Check sheet for the modelled part. Datum: model origin and axes. Units: mm. Face numbers are marked on the shaded views. A direction names the side the tool comes from. Give positions to 0.01 mm unless a question says otherwise; leave off trailing zeros. Order: outer loops, then holes, each group sorted by start corner. A loop starts at its lowest first (then second) coordinate and runs counter-clockwise, first axis right, second up.
Item 1: Access from +Z, -Z, +X, -X, +Y, -Y to the whole of each face (thin tool, end or side, straight path). Record for the marked faces 5, 6, 7, 8 and 9.
Item 2: Sectioned sample at D-D on y = -6. Record the boundary of the cut face in (x, z).
Item 3: Sectioned sample at A-A on y = -8.5. Record the boundary of the cut face in (x, z), and give its area (3 significant figures).
Item 4: Gauge pin test, flat ends, axial feed: P1, Ø6.5, axis at x = -14.5, z = 1, coming from the +Y side; P2, Ø2.5, axis at x = 0, z = -6, coming from the -Y side; P3, Ø6.5, axis at y = -4, z = -0.5, coming from the +X side; P4, Ø0.6, axis at y = 1, z = -4.5, coming from the -X side. Record the tip position at first contact, or that the pin passes through.
Item 5: Material ranges on line 1 along X through (y, z) = (-9.15, 0); line 2 along Z through (x, y) = (0, 0.45); line 3 along Y through (x, z) = (11.5, 1.5), recorded low to high.
Item 6: Sectioned sample at B-B on z = 0. Record the boundary of the cut face in (x, y), and give its area (3 significant figures).
Item 7: Release check for a two-part mould opening along X. For the marked faces 1, 2, 3 and 4 record: released by +X, released by -X, zero draft, split by the parting line, or undercut.
Item 8: Sectioned sample at C-C on x = 0. Record the boundary of the cut face in (y, z).
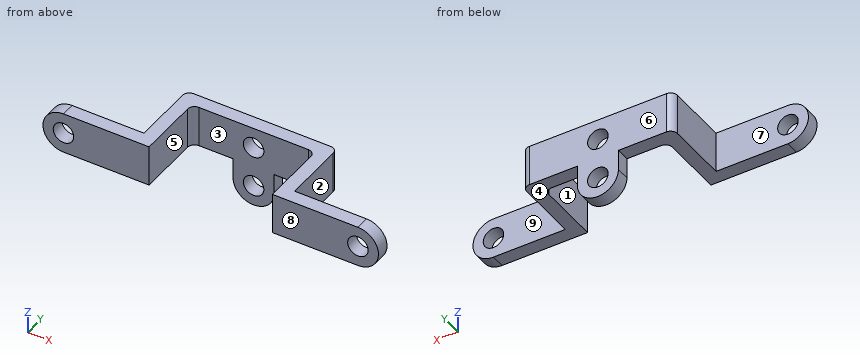
Autodesk Inventor part; units mm, degrees
ref_plane "YZ Plane" through (0, 0, 0) normal (1, 0, 0) x (0, 1, 0)
ref_plane "XZ Plane" through (0, 0, 0) normal (0, 1, 0) x (-1, 0, 0)
ref_plane "XY Plane" through (0, 0, 0) normal (0, 0, 1) x (1, 0, 0)
sketch "Sketch1" plane through (0, 0, 0) normal (0, 1, 0) x (-1, 0, 0)
  line L0 (11, 3) -> (-11, 3)
  line L1 (-11, 3) -> (-11, -3)
  line L2 (-11, -3) -> (11, -3)
  line L3 (11, -3) -> (11, 3)
  line L4 (11, 3) -> (-11, -3) construction
  line L5 (-11, 3) -> (11, -3) construction
  point P0 (0, 0)
  dimension "d0" = 22
  dimension "d1" = 6
extrude "Extrusion1" add sketch "Sketch1" along normal blind 2
sketch "Sketch2" plane through (0, 0, 0) normal (0, -1, 0) x (1, 0, 0)
  line L0 (11, -3) -> (-11, -3)
  line L1 (-11, 3) -> (-9, 3)
  line L2 (-9, 3) -> (-9, -3)
  line L3 (-9, -3) -> (-11, -3)
  line L4 (-11, -3) -> (-11, 3)
  line L5 (11, 3) -> (9, 3)
  line L6 (9, 3) -> (9, -3)
  line L7 (9, -3) -> (11, -3)
  line L8 (11, -3) -> (11, 3)
  point P0 (0, 0)
  dimension "d4" = 2
  dimension "d5" = 2
extrude "Extrusion2" add sketch "Sketch2" along normal blind 10
sketch "Sketch3" plane through (11, 2, 3) normal (1, 0, 0) x (0, 0, -1)
  line L0 (0, -12) -> (6, -12)
  line L1 (6, -12) -> (6, -10)
  line L2 (6, -10) -> (0, -10)
  line L3 (0, -10) -> (0, -12)
  point P0 (3, -2)
  dimension "d8" = 6
  dimension "d9" = 2
sketch "Sketch4" plane through (-11, 2, -3) normal (-1, 0, 0) x (0, 0, 1)
  line L0 (0, -12) -> (6, -12)
  line L1 (6, -12) -> (6, -10)
  line L2 (6, -10) -> (0, -10)
  line L3 (0, -10) -> (0, -12)
  point P0 (3, -2)
  dimension "d10" = 6
  dimension "d11" = 2
extrude "Extrusion3" add sketch "Sketch4" along normal blind 14
extrude "Extrusion4" add sketch "Sketch3" along normal blind 14
sketch "Sketch5" plane through (11, -8, 3) normal (0, 1, 0) x (1, 0, 0)
  line L0 (0, 0) -> (14, 0)
  line L1 (14, 6) -> (14, 0)
  line L2 (0, 6) -> (14, 6)
  line L3 (14, 3) -> (10.5, 3)
  circle A0 centre (10.5, 3) radius 3.5
  line L4 (12.3028, 6) -> (14, 6)
  line L5 (14, 3) -> (14, 6)
  line L6 (14, 3) -> (14, 0)
  line L7 (14, 0) -> (12.3028, 0)
  point P0 (-11, 3)
  dimension "d16" = 3.5
sketch "Sketch6" plane through (-11, -8, 3) normal (0, 1, 0) x (1, 0, 0)
  line L0 (0, 6) -> (0, 0)
  line L1 (0, 6) -> (-14, 6)
  line L2 (-14, 0) -> (-14, 6)
  line L3 (0, 0) -> (-14, 0)
  line L4 (-14, 3) -> (-10.5, 3)
  circle A0 centre (-10.5, 3) radius 3.5
  line L5 (-12.3028, 0) -> (-14, 0)
  line L6 (-14, 0) -> (-14, 3)
  line L7 (-14, 6) -> (-14, 3)
  line L8 (-14, 6) -> (-12.3028, 6)
  point P0 (11, 3)
  point P1 (0, -0.5)
  dimension "d17" = 3.5
extrude "Extrusion5" cut sketch "Sketch5" against normal blind 2 contours A0 L1 L0 | A0 L2 L1
extrude "Extrusion6" cut sketch "Sketch6" against normal blind 2 contours A0 L2 L1 | L3 L2 A0
sketch "Sketch7" plane through (11, -8, 3) normal (0, 1, 0) x (1, 0, 0)
  arc A0 (12.3028, 0) -> (12.3028, 6) centre (10.5, 3) ccw
  circle A1 centre (10.5, 3) radius 1.5
  point P0 (-11, 3)
  dimension "d22" = 3
extrude "Extrusion7" cut sketch "Sketch7" against normal blind 2
sketch "Sketch8" plane through (-11, -8, 3) normal (0, 1, 0) x (1, 0, 0)
  arc A0 (-12.3028, 6) -> (-12.3028, 0) centre (-10.5, 3) ccw
  circle A1 centre (-10.5, 3) radius 1.5
  point P0 (11, 3)
  dimension "d25" = 3
extrude "Extrusion8" cut sketch "Sketch8" against normal blind 2
fillet "Fillet1" radius 1 4 edges at (11, 2, 0) (-11, 2, 0) (9, 0, 0) (-9, 0, 0)
sketch "Sketch9" plane through (0, 2, 0) normal (0, 1, 0) x (1, 0, 0)
  line L0 (-10, -3) -> (10, -3)
  line L1 (10, 3) -> (-10, 3)
  line L2 (0, -3) -> (0, 0)
  circle A0 centre (0, 0) radius 1.5
  point P0 (0, 0)
  dimension "d29" = 3
  dimension "d30" = 3
extrude "Extrusion9" cut sketch "Sketch9" against normal blind 2
sketch "Sketch10" plane through (0, 2, 0) normal (0, 1, 0) x (1, 0, 0)
  circle A0 centre (0, 0) radius 1.5
  line L0 (10, 3) -> (-10, 3)
  line L1 (0, 0) -> (0, 6)
  circle A1 centre (0, 6) radius 1.5
  line L2 (0, 6) -> (0, 9)
  line L3 (-3.5, 5) -> (-3.5, 3)
  line L4 (3.5, 5) -> (3.5, 3)
  arc A2 (3.5, 5) -> (-3.5, 5) centre (0, 5) ccw
  line L5 (-3.5, 3) -> (3.5, 3)
  point P0 (0, 0)
  dimension "d33" = 6
  dimension "d34" = 3
  dimension "d35" = 3
extrude "Extrusion10" add sketch "Sketch10" against normal blind 2 contours L0 L3 A2 L2 A1 L1 | L1 A1 L2 A2 L4 L0
sketch "Sketch11" plane through (11, -8, 3) normal (0, 1, 0) x (1, 0, 0)
  arc A0 (12.3028, 0) -> (12.3028, 6) centre (10.5, 3) ccw
  line L0 (0, 6) -> (12.3028, 6)
  line L1 (0, 0) -> (12.3028, 0)
  circle A1 centre (10.5, 3) radius 3
  line L2 (10.5, 0) -> (12.3028, 0)
  line L3 (10.5, 6) -> (12.3028, 6)
  arc A2 (12.3028, 0) -> (12.3028, 6) centre (10.5, 3) ccw
  point P0 (-11, 3)
extrude "Extrusion11" cut sketch "Sketch11" against normal blind 2 contours L1 A1 L0 A0
sketch "Sketch12" plane through (-11, -8, 3) normal (0, 1, 0) x (1, 0, 0)
  arc A0 (-12.3028, 6) -> (-12.3028, 0) centre (-10.5, 3) ccw
  line L0 (0, 0) -> (-12.3028, 0)
  line L1 (0, 6) -> (-12.3028, 6)
  circle A1 centre (-10.5, 3) radius 3
  line L2 (-12.3028, 0) -> (-10.5, 0)
  line L3 (-12.3028, 6) -> (-10.5, 6)
  arc A2 (-12.3028, 6) -> (-12.3028, 0) centre (-10.5, 3) ccw
  point P0 (11, 3)
extrude "Extrusion12" cut sketch "Sketch12" against normal blind 2 contours L1 A1 L0 A0
sketch "Sketch13" plane through (0, 2, 0) normal (0, 1, 0) x (1, 0, 0)
  circle A0 centre (0, 6) radius 1.5
  line L0 (3.5, 3) -> (3.5, 5)
  arc A1 (3.5, 5) -> (-3.5, 5) centre (0, 5) ccw
  line L1 (-3.5, 5) -> (-3.5, 3)
  line L2 (-3.5, 3) -> (-10, 3)
  circle A2 centre (0, 6) radius 1.5
  circle A3 centre (0, 6) radius 3
  line L3 (-3.5, 3) -> (3.5, 3)
  line L4 (3.5, 3) -> (3.5, 5)
  line L5 (-3.5, 3) -> (-3.5, 5)
  line L6 (-3, 6) -> (-3, 3)
  line L7 (3, 6) -> (3, 3)
  line L8 (-3, 3) -> (-3.5, 3)
  line L9 (3, 3) -> (3.5, 3)
  arc A4 (3.5, 5) -> (-3.5, 5) centre (0, 5) ccw
  dimension "d44" = 3
  dimension "d45" = 6
extrude "Extrusion13" cut sketch "Sketch13" against normal blind 2 contours L3 L7 A3 A1 L0 | A3 A1 | A3 L6 L3 L1 A1 picked at (-2.1113, 7.1747)
sketch "Sketch14" plane through (0, 2, 0) normal (0, 1, 0) x (1, 0, 0)
  arc A0 (-3, 6) -> (3, 6) centre (0, 6) ccw
  circle A1 centre (0, 6) radius 3
  circle A2 centre (0, 6) radius 1.5
  dimension "d48" = 3
extrude "Extrusion14" add sketch "Sketch14" against normal blind 2
properties part number "tahlo6"
Report:
1. face 5: +Z, -Z, -Y
1. face 6: +Z, -Z, +X, -X, +Y
1. face 7: +Z, -Z, -X, +Y
1. face 8: +Z, -Z, +X, -X, -Y
1. face 9: +Z, -Z, +X, +Y
2. outline: (-11, -3) - (-9, -3) - (-9, 3) - (-11, 3) - close; (9, -3) - (11, -3) - (11, 3) - (9, 3) - close
3. outline: (-21.5, -3) - (-9, -3) - (-9, 3) - (-21.5, 3) arc R3 ccw to start; (9, -3) - (21.5, -3) arc R3 ccw to (21.5, 3) - (9, 3) - close; hole circle Ø3 at (-21.5, 0); hole circle Ø3 at (21.5, 0)
3. area: 164 mm2
4. P1: stops at y = -8
4. P2: passes through
4. P3: stops at x = 11
4. P4: stops at x = -3
5. line 1: x = -24.5 to -23, -20 to -9, 9 to 20, 23 to 24.5
5. line 2: z = -9 to -7.5, -4.5 to -1.5, 1.5 to 3
5. line 3: y = -10 to -8
6. outline: (-24.5, -10) - (-23, -10) - (-23, -8) - (-24.5, -8) - close; (-20, -10) - (-9, -10) - (-9, -1) arc R1 cw to (-8, 0) - (-1.5, 0) - (-1.5, 2) - (-10, 2) arc R1 ccw to (-11, 1) - (-11, -8) - (-20, -8) - close; (1.5, 0) - (8, 0) arc R1 cw to (9, -1) - (9, -10) - (20, -10) - (20, -8) - (11, -8) - (11, 1) arc R1 ccw to (10, 2) - (1.5, 2) - close; (23, -10) - (24.5, -10) - (24.5, -8) - (23, -8) - close
6. area: 120 mm2
7. face 1: undercut
7. face 2: released by +X
7. face 3: undercut
7. face 4: zero draft
8. outline: (0, -9) - (2, -9) - (2, -7.5) - (0, -7.5) - close; (0, -4.5) - (2, -4.5) - (2, -1.5) - (0, -1.5) - close; (0, 1.5) - (2, 1.5) - (2, 3) - (0, 3) - close
